Check sheet for the modelled part. Datum: model origin and axes. Units: mm. A direction names the side the tool comes from. Round coordinates to 2 decimals unless told otherwise and drop trailing zeros. Write each loop counter-clockwise with the first axis right and the second up, starting at its lowest first coordinate (ties: lowest second). Pieces come first, ordered by that corner, then holes.
Item 1: Cross-section at A-A on x = 17.78. Enter the section's corners in (y, z) (3 decimals).
Item 2: Cross-section at C-C on z = -41. Enter the section's corners in (x, y), plus the area to 3 significant figures.
Item 3: Release check for a two-part mould opening along Z. For faces 1 (the flat face through (30, 3, -39.243)), 2 (the flat face through (127, 7.62, -5)), 3 (the cylindrical face through (1.449, 2.576, -64.512)), 4 (the flat face through (65, 3, 0)) record: +Z half, -Z half, draft (parallel to the pull), parting line (faces both ways), or undercut.
Item 4: Material ranges on line 1 (X direction, y = 3.35, z = -25.4) (3 decimals); line 2 (Y direction, x = 104, z = -27); line 3 (X direction, y = 3, z = -41.5), recorded low to high.
Item 5: Go/stop test with flat-tipped pins: pin 1 Ø7 at (x, z) = (18.5, -40.5) entering from +Y; pin 2 Ø3 at (x, z) = (17.78, -40.64) entering from +Y. Record where each tip stops, or that it passes through.
Item 6: Cross-section at D-D on x = 70. Enter the section's corners in (y, z), plus the area to 3 significant figures.
Item 7: Tool access check on faces 5 (the flat face through (30, 3, -26.797)), 6 (the cylindrical face through (16.56, 3.2, -22.47)), 7 (the flat face through (65, 0, -33)). Record the directions out of +Z, -Z, +X, -X, +Y, -Y that give a thin tool (end or side, any length) a straight path to the whole face; none if there is none.
Item 8: Cross-section at B-B on y = 3. Enter the section's corners in (x, z) (3 decimals), plus the area to 3 significant figures.
from build123d import *

# Parameters (mm, degrees)
SKETCH1_W           = 121.92
SKETCH1_H           = 66.04
BOSS_EXTRUDE1_DEPTH = 5.08
FILLET1_R           = 5.08
CUT_EXTRUDE2_REACH  = 140.75
SKETCH2_R           = 1.7526
SKETCH2_W           = 6.096
SKETCH2_H           = 12.446
SKETCH3_R           = 3.175
CUT_EXTRUDE3_DEPTH  = 3.81
CUT_EXTRUDE4_REACH  = 140.709
SKETCH4_R           = 1.9812
SKETCH8_W           = 15.24
SKETCH8_H           = 66.04
BOSS_EXTRUDE2_DEPTH = 5.08
FILLET4_R           = 5.08
SKETCH5_R           = 2.286
BOSS_EXTRUDE3_DEPTH = 2.54


with BuildPart() as part:
    # Sketch1 → Boss-Extrude1 (new body)
    with BuildSketch(Plane(origin=(0, 0, 0), x_dir=(1, 0, 0), z_dir=(0, 1, 0))):
        with Locations((60.96, 33.02)):
            Rectangle(SKETCH1_W, SKETCH1_H)
    extrude(amount=BOSS_EXTRUDE1_DEPTH)

    # Fillet1
    fillet1_edges = [part.edges().sort_by_distance(p)[0] for p in [
        (0, 2.54, -66.04),
        (121.92, 2.54, -66.04),
        (121.92, 2.54, 0),
        (0, 2.54, 0),
    ]]
    fillet(fillet1_edges, radius=FILLET1_R)

    # Sketch2 → Cut-Extrude2 (cut, up to next)
    with BuildSketch(Plane(origin=(0, 5.08, 0), x_dir=(1, 0, 0), z_dir=(0, 1, 0)), mode=Mode.PRIVATE) as cut_extrude2_sk1:
        with Locations(Location((30.48, 47.2694, 0), (0, 0, 270))):
            Circle(SKETCH2_R)
    cut_extrude2_tool1 = extrude(cut_extrude2_sk1.sketch, amount=-CUT_EXTRUDE2_REACH, mode=Mode.PRIVATE) & part.part
    # Sketch2 → Cut-Extrude2 (cut, up to next)
    with BuildSketch(Plane(origin=(0, 5.08, 0), x_dir=(1, 0, 0), z_dir=(0, 1, 0)), mode=Mode.PRIVATE) as cut_extrude2_sk2:
        with Locations(Location((30.48, 18.7706, 0), (0, 0, 90))):
            Circle(SKETCH2_R)
    cut_extrude2_tool2 = extrude(cut_extrude2_sk2.sketch, amount=-CUT_EXTRUDE2_REACH, mode=Mode.PRIVATE) & part.part
    # Sketch2 → Cut-Extrude2 (cut, up to next)
    with BuildSketch(Plane(origin=(0, 5.08, 0), x_dir=(1, 0, 0), z_dir=(0, 1, 0)), mode=Mode.PRIVATE) as cut_extrude2_sk3:
        with Locations((30.48, 33.02)):
            Rectangle(SKETCH2_W, SKETCH2_H)
    cut_extrude2_tool3 = extrude(cut_extrude2_sk3.sketch, amount=-CUT_EXTRUDE2_REACH, mode=Mode.PRIVATE) & part.part
    add(cut_extrude2_tool1.solids().sort_by_distance((30.48, 5.08, -47.2694))[0], mode=Mode.SUBTRACT)
    add(cut_extrude2_tool2.solids().sort_by_distance((30.48, 5.08, -18.7706))[0], mode=Mode.SUBTRACT)
    add(cut_extrude2_tool3.solids().sort_by_distance((30.48, 5.08, -33.02))[0], mode=Mode.SUBTRACT)

    # Sketch3 → Cut-Extrude3 (cut)
    with BuildSketch(Plane(origin=(0, 5.08, 0), x_dir=(1, 0, 0), z_dir=(0, 1, 0))):
        with Locations(Location((17.78, 40.64, 0), (0, 0, 270))):
            Circle(SKETCH3_R)
        with Locations(Location((17.78, 25.4, 0), (0, 0, 270))):
            Circle(SKETCH3_R)
    extrude(amount=-CUT_EXTRUDE3_DEPTH, mode=Mode.SUBTRACT)

    # Sketch4 → Cut-Extrude4 (cut, up to next)
    with BuildSketch(Plane(origin=(0, 1.27, 0), x_dir=(1, 0, 0), z_dir=(0, 1, 0)), mode=Mode.PRIVATE) as cut_extrude4_sk1:
        with Locations(Location((17.78, 40.64, 0), (0, 0, 270))):
            Circle(SKETCH4_R)
    cut_extrude4_tool1 = extrude(cut_extrude4_sk1.sketch, amount=-CUT_EXTRUDE4_REACH, mode=Mode.PRIVATE) & part.part
    # Sketch4 → Cut-Extrude4 (cut, up to next)
    with BuildSketch(Plane(origin=(0, 1.27, 0), x_dir=(1, 0, 0), z_dir=(0, 1, 0)), mode=Mode.PRIVATE) as cut_extrude4_sk2:
        with Locations(Location((17.78, 25.4, 0), (0, 0, 270))):
            Circle(SKETCH4_R)
    cut_extrude4_tool2 = extrude(cut_extrude4_sk2.sketch, amount=-CUT_EXTRUDE4_REACH, mode=Mode.PRIVATE) & part.part
    add(cut_extrude4_tool1.solids().sort_by_distance((17.78, 1.27, -40.64))[0], mode=Mode.SUBTRACT)
    add(cut_extrude4_tool2.solids().sort_by_distance((17.78, 1.27, -25.4))[0], mode=Mode.SUBTRACT)

    # Sketch8 → Boss-Extrude2 (add)
    with BuildSketch(Plane.XZ):
        with Locations((124.46, -33.02)):
            Rectangle(SKETCH8_W, SKETCH8_H)
    extrude(amount=-BOSS_EXTRUDE2_DEPTH)

    # Fillet4
    fillet4_edges = [part.edges().sort_by_distance(p)[0] for p in [
        (132.08, 2.54, 0),
        (132.08, 2.54, -66.04),
    ]]
    fillet(fillet4_edges, radius=FILLET4_R)

    # Sketch5 → Boss-Extrude3 (add)
    with BuildSketch(Plane(origin=(0, 5.08, 0), x_dir=(1, 0, 0), z_dir=(0, 1, 0))):
        with Locations(Location((5.08, 60.96, 0), (0, 0, 90))):
            Circle(SKETCH5_R)
        with Locations(Location((127, 60.96, 0), (0, 0, 90))):
            Circle(SKETCH5_R)
        with Locations(Location((127, 5.08, 0), (0, 0, 90))):
            Circle(SKETCH5_R)
        with Locations(Location((5.08, 5.08, 0), (0, 0, 90))):
            Circle(SKETCH5_R)
    extrude(amount=BOSS_EXTRUDE3_DEPTH)


solid = part.part
Response values:
1. outline: (0, -66.04) - (5.08, -66.04) - (5.08, -43.815) - (1.27, -43.815) - (1.27, -42.621) - (0, -42.621) - close; (0, -38.659) - (1.27, -38.659) - (1.27, -37.465) - (5.08, -37.465) - (5.08, -28.575) - (1.27, -28.575) - (1.27, -27.381) - (0, -27.381) - close; (0, -23.419) - (1.27, -23.419) - (1.27, -22.225) - (5.08, -22.225) - (5.08, 0) - (0, 0) - close
2. outline: (0, 0) - (15.83, 0) - (15.83, 1.27) - (14.63, 1.27) - (14.63, 5.08) - (0, 5.08) - close; (19.73, 0) - (132.08, 0) - (132.08, 5.08) - (20.93, 5.08) - (20.93, 1.27) - (19.73, 1.27) - close
2. area: 642 mm2
3. face 1: undercut
3. face 2: draft
3. face 3: -Z half
3. face 4: +Z half
4. line 1: x = 0 to 14.605, 20.955 to 132.08
4. line 2: y = 0 to 5.08
4. line 3: x = 0 to 14.72, 20.84 to 132.08
5. pin 1: stops at y = 5.08
5. pin 2: passes through
6. outline: (0, -66.04) - (5.08, -66.04) - (5.08, 0) - (0, 0) - close
6. area: 335 mm2
7. face 5: +Y, -Y
7. face 6: +Y
7. face 7: +Z, -Z, +X, -X, -Y
8. outline: (0, -60.96) arc R5.08 ccw to (5.08, -66.04) - (127, -66.04) arc R5.08 ccw to (132.08, -60.96) - (132.08, -5.08) arc R5.08 ccw to (127, 0) - (5.08, 0) arc R5.08 ccw to (0, -5.08) - close; hole circle Ø6.35 at (17.78, -40.64); hole circle Ø6.35 at (17.78, -25.4); hole (27.432, -39.243) - (33.528, -39.243) - (33.528, -26.797) - (27.432, -26.797) - close; hole circle Ø3.505 at (30.48, -47.269); hole circle Ø3.505 at (30.48, -18.771)
8. area: 8,540 mm2
